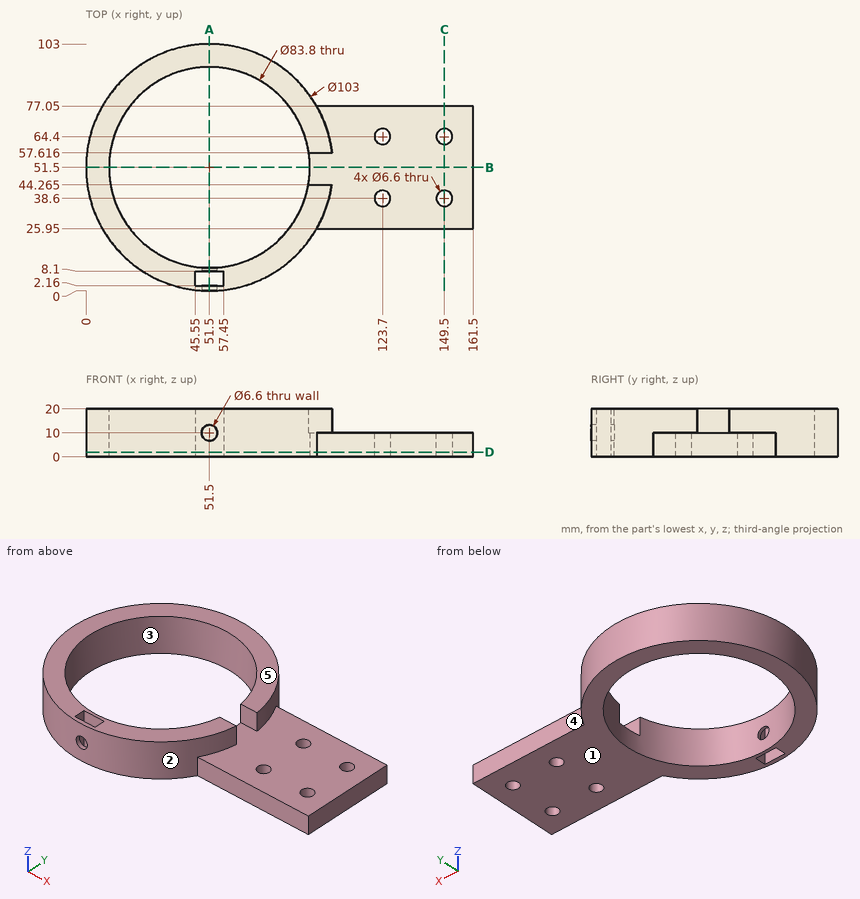
Print and shaded views of the part. All mm, measured from the part's lowest x, y and z. A direction names the side the tool comes from. Round coordinates to 2 decimals unless told otherwise and drop trailing zeros. Write each loop counter-clockwise with the first axis right and the second up, starting at its lowest first coordinate (ties: lowest second). Pieces come first, ordered by that corner, then holes. Notation, with made-up numbers: (78.5, -27) - (103.5, -27) arc R19 cw to (103.5, 0) - close; hole circle Ø10 at (-14.5, 48). An arc over 180 degrees is marked (long way). Write each question's results on one line, items separated by ' | '. Start each with the question number.
Item 1: Saw through at A-A (x = 51.5). Write the cut outline in (y, z).
Item 2: Which spindle directions (+Z, -Z, +X, -X, +Y, -Y) get a long thin tool onto all of the face, cutting with end or side? Do the marked faces 4 and 5. Say none if no direction does.
Item 3: Saw through at C-C (x = 149.5). Write the cut outline in (y, z), and give its area (3 significant figures).
Item 4: Mould opens along Y. For the marked faces 1, 2 and 3 say: pulls with the +Y half, pulls with the -Y half, needs draft (parallel to the pull), parting line crosses it, or undercut.
Item 5: Wall check: L1, parallel to Y at x = 123.7, z = 7.5; L2, parallel to Z at x = 124.5, y = 33; L3, parallel to Y at x = 24.5, z = 15.75 (1 decimal). Give the ranges that are in metal, low to high. Write a range as [from, to].
Item 6: Drop flat-ended pins along their axis: P1, Ø12, axis at y = 32.5, z = 8, coming from the -X side; P2, Ø9.5, axis at x = 52.5, z = 13, coming from the +Y side; P3, Ø2, axis at x = 100, z = 8, coming from the +Y side; P4, Ø6, axis at x = 49.5, z = 7, coming from the -Y side. Give the stop position or say it passes through.
Item 7: Saw through at B-B (y = 51.5). Write the cut outline in (x, z), and give its area (3 significant figures).
Item 8: Saw through at D-D (z = 2). State how many separate pieces and enclosed holes the cut face has, and give its area (3 significant figures).
Results are:
1) outline: (0, 0) - (2.16, 0) - (2.16, 6.7) - (0, 6.7) - close; (0, 13.3) - (2.16, 13.3) - (2.16, 20) - (0, 20) - close; (8.1, 0) - (9.6, 0) - (9.6, 6.7) - (8.1, 6.7) - close; (8.1, 13.3) - (9.6, 13.3) - (9.6, 20) - (8.1, 20) - close; (93.4, 0) - (103, 0) - (103, 20) - (93.4, 20) - close
2) face 4: +Z, -Z, +X, +Y | face 5: +Z, +X, -X, +Y, -Y
3) outline: (25.95, 0) - (35.3, 0) - (35.3, 10) - (25.95, 10) - close; (41.9, 0) - (61.1, 0) - (61.1, 10) - (41.9, 10) - close; (67.7, 0) - (77.05, 0) - (77.05, 10) - (67.7, 10) - close | area: 379 mm²
4) face 1: needs draft | face 2: parting line crosses it | face 3: undercut
5) L1: y = [25.95, 35.3], [41.9, 61.1], [67.7, 77.05] | L2: z = [0, 10] | L3: y = [7.6, 19.5], [83.5, 95.4]
6) P1: stops at x = 1.67 | P2: stops at y = 103 | P3: stops at y = 77.05 | P4: stops at y = 0
7) outline: (0, 0) - (9.6, 0) - (9.6, 20) - (0, 20) - close; (93.4, 0) - (161.5, 0) - (161.5, 10) - (93.4, 10) - close | area: 873 mm²
8) separate pieces: 1 | enclosed holes: 6 | area: 5,710 mm²
